Here's how the part is built. I have some questions about the finished solid (model axes, mm). Face numbers are marked on the shaded views. A direction names the side the tool comes from. Coordinates: 2 decimals unless noted, no trailing zeros.
Item 1: For the marked faces 4 and 5, which set-ups out of +Z, -Z, +X, -X, +Y, -Y let a thin tool reach every point of the face, with its end or its side?
Item 2: Please list where these lines run through material, in increasing order: line 1 (X direction, y = 32.5, z = 2.5); line 2 (X direction, y = 7.5, z = 36); line 3 (Y direction, x = -79, z = -26).
Item 3: I'm going to push flat-ended pins straight in: P1, Ø8, axis at x = 10.5, y = -12, coming from the -Z side; P2, Ø4, axis at x = 38.5, y = -10, coming from the +Z side; P3, Ø12, axis at x = 79.5, y = -30.5, coming from the +Z side. Where does each tip first touch, or does it pass through?
Item 4: If we mould it in two halves opening along X, with no side actions, what happens to the marked faces 1, 2 and 3? For each: pulls with the +X half, pulls with the -X half, needs draft (parallel to the pull), parting line crosses it, or undercut.
from build123d import *

# Parameters (mm, degrees)
SKETCH5_R           = 15
BOSS_EXTRUDE1_DEPTH = 115
SKETCH6_R           = 40
BOSS_EXTRUDE2_DEPTH = 40
BOSS_EXTRUDE3_START = -40
SKETCH7_R           = 40
BOSS_EXTRUDE3_DEPTH = 40
FILLET2_R           = 5
CHAMFER1_SIZE       = 5


with BuildPart() as part:
    # Sketch5 → Boss-Extrude1 (new, symmetric)
    with BuildSketch(Plane(origin=(0, 0, 0), x_dir=(0, 0, -1), z_dir=(1, 0, 0))):
        Circle(SKETCH5_R)
    extrude(amount=BOSS_EXTRUDE1_DEPTH, both=True)

    # Sketch6 → Boss-Extrude2 (add)
    with BuildSketch(Plane(origin=(115, 0, 0), x_dir=(0, 0, -1), z_dir=(1, 0, 0))):
        Circle(SKETCH6_R)
    extrude(amount=-BOSS_EXTRUDE2_DEPTH)

    # Sketch7 → Boss-Extrude3 (add)
    with BuildSketch(Plane.ZY.offset(115).offset(BOSS_EXTRUDE3_START)):
        with Locations(Location((0, 0, 0), (0, 0, 180))):
            Circle(SKETCH7_R)
    extrude(amount=BOSS_EXTRUDE3_DEPTH)

    # Sketch9 → Revolve1 (revolve)
    with BuildSketch(Plane.XY, mode=Mode.PRIVATE) as revolve1_sk:
        with BuildLine():
            Line((-75, 15), (75, 15))
            ThreePointArc((75, 15), (0, 20), (-75, 15))
        make_face()
    revolve(revolve1_sk.sketch.rotate(Axis((0, 0, 0), (-1, 0, 0)), 90), axis=Axis((0, 0, 0), (-1, 0, 0)))

    # Fillet2
    fillet2_edges = [part.edges().sort_by_distance(p)[0] for p in [
        (-75, 0, 15),
        (75, 0, 15),
    ]]
    fillet(fillet2_edges, radius=FILLET2_R)

    # Chamfer1
    chamfer1_edges = [part.edges().sort_by_distance(p)[0] for p in [
        (-75, 0, 40),
        (-115, 0, 40),
        (75, 0, 40),
        (115, 0, 40),
    ]]
    chamfer(chamfer1_edges, length=CHAMFER1_SIZE)


solid = part.part
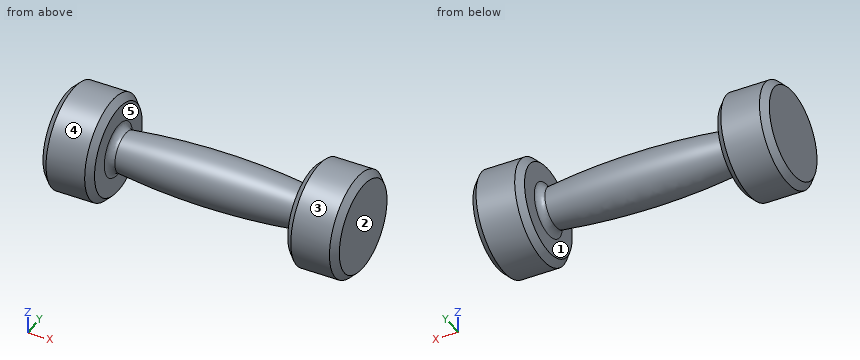
Answer:
1. face 4: +X, -X
1. face 5: none
2. line 1: x = -115 to -75, 75 to 115
2. line 2: x = -113.23 to -76.77, 76.77 to 113.23
2. line 3: y = -29.07 to 29.07
3. P1: stops at z = -18.23
3. P2: stops at z = 16.9
3. P3: stops at z = 31.6
4. face 1: undercut
4. face 2: pulls with the +X half
4. face 3: needs draft
